```python
from build123d import *

# Parameters (mm, degrees)
SKETCH003_R   = 1.35
EXTRUDE_DEPTH = 30


with BuildPart() as hole_cut:
    # Sketch003 → Extrude (new body, symmetric)
    with BuildSketch(Plane.XY):
        with Locations((42.497118, 42.497118)):
            Circle(SKETCH003_R)
        with Locations((0, 60.1)):
            Circle(SKETCH003_R)
        with Locations((-42.497118, 42.497118)):
            Circle(SKETCH003_R)
        with Locations((-60.1, 0)):
            Circle(SKETCH003_R)
        with Locations((-42.497118, -42.497118)):
            Circle(SKETCH003_R)
        with Locations((0, -60.1)):
            Circle(SKETCH003_R)
        with Locations((42.497118, -42.497118)):
            Circle(SKETCH003_R)
        with Locations((60.1, 0)):
            Circle(SKETCH003_R)
    extrude(amount=EXTRUDE_DEPTH, both=True)


with BuildPart() as bearing_inner_race_upper:
    # Sketch → Revolve (revolve)
    with BuildSketch(Plane.XZ):
        with BuildLine():
            ThreePointArc((-77.6, 0), (-78.055778, 1.407125), (-79.25, 2.279803))
            Line((-79.25, 2.279803), (-79.25, 6))
            Line((-79.25, 6), (-42.6, 6))
            Line((-42.6, 6), (-42.6, 0))
            Line((-77.6, 0), (-42.6, 0))
        make_face()
    revolve(axis=Axis((0, 0, 0), (0, 0, 1)))

    # Cut: cut hole cut
    add(hole_cut.part, mode=Mode.SUBTRACT)


solid = bearing_inner_race_upper.part
```
The model under review builds one solid part; all positions refer to its coordinate system, in mm. Coordinates: 2 decimals unless noted, no trailing zeros. Answer in a Markdown table with one row per item. Add a question column.
Item 1: We need section A-A on z = 5. Give the number of separate pieces and of enclosed holes in the cut face, plus the area to 3 significant figures.
Item 2: Clearance check with flat-ended pins moving along their axes: pin 1 (1.5 mm diameter, centred on y = 15.5, z = 5, fed in from +X); pin 2 (1.6 mm diameter, centred on x = 60.1, y = 0, fed in from -Z); pin 3 (1 mm diameter, centred on y = 17.5, z = 4.5, fed in from -X); pin 4 (1.5 mm diameter, centred on x = 3, z = 1, fed in from -Y). State where each tip first meets the part, or that it passes through.
Item 3: To check wall thickness, follow probe 1 along Y at (x, z) = (0, 3.8); probe 2 along Y at (x, z) = (23, 5.3); probe 3 along X at (y, z) = (-17.5, 1.95). State the ranges of each line that lie inside material, in increasing order.
Item 4: Mouldability with a two-part tool opening along Y and no side actions: class faces 1 (the cylindrical face through (-40.63, -12.8, 2.96)), 2 (the cylindrical face through (10.317, -78.576, 4.166)), 3 (the flat face through (-34, 34, 6)) as +Y half, -Y half, draft (parallel to the pull), parting line (faces both ways), or undercut.
Final values:
| question | item | result |
|---|---|---|
| 1 | separate pieces | 1 |
| 1 | enclosed holes | 9 |
| 1 | area | 14,000 mm2 |
| 2 | pin 1 | stops at x = 77.87 |
| 2 | pin 2 | passes through |
| 2 | pin 3 | stops at x = -77.41 |
| 2 | pin 4 | stops at y = -78.3 |
| 3 | probe 1 | y = -79.25 to -61.45, -58.75 to -42.6, 42.6 to 58.75, 61.45 to 79.25 |
| 3 | probe 2 | y = -75.84 to -35.86, 35.86 to 75.84 |
| 3 | probe 3 | x = -76.63 to -38.84, 38.84 to 76.63 |
| 4 | face 1 | undercut |
| 4 | face 2 | parting line |
| 4 | face 3 | draft |
